from build123d import *

# Parameters (mm, degrees)
F1_DEPTH        = 1
F3_DEPTH        = 0.5
F5_DEPTH        = 5
F10_D           = 2
F10_DEPTH       = 5
F10_TIP         = 0.600860619
F10_ON_F7_D     = 2
F10_ON_F7_DEPTH = 5
F10_ON_F7_TIP   = 0.600860619
F10_ON_F8_D     = 2
F10_ON_F8_DEPTH = 5
F10_ON_F8_TIP   = 0.600860619
F10_ON_F9_D     = 2
F10_ON_F9_DEPTH = 5
F10_ON_F9_TIP   = 0.600860619


# Not quite as in the source:
# - ends of sketch curves that miss each other by under 0.0002 mm in the source are joined


with BuildPart() as f1:
    # F0 (on Top) → F1 (new body)
    with BuildSketch(Plane.XY):
        with BuildLine():
            ThreePointArc((87.5, -67.5), (100, 0), (87.5, 67.5))
            ThreePointArc((87.5, 67.5), (0, 75), (-87.5, 67.5))
            ThreePointArc((-87.5, 67.5), (-100, 0), (-87.5, -67.5))
            ThreePointArc((-87.5, -67.5), (0, -75), (87.5, -67.5))
        make_face()
    extrude(amount=F1_DEPTH)

    # F2 (on face) → F3 (cut)
    with BuildSketch(Plane(origin=(0, 0, 0), x_dir=(1, 0, 0), z_dir=(0, 0, -1))):
        Polygon((59.9405638027, -1.5313209672), (59.9405638027, -3.714e-05), (59.9405638027, 1.5331036891), (59.6300730728, 6.1295549733), (58.7212563071, 12.0819890983), (57.2441969375, 17.8245820004), (55.2293497966, 23.3313356518), (52.7045699138, 28.5721666207), (49.7021691234, 33.5132774711), (46.2529736583, 38.1275559743), (42.3840957472, 42.3849186981), (38.126361623, 46.2537966092), (33.5117117195, 49.7033634747), (28.5691152675, 52.705764265), (23.3301413005, 55.2305441479), (17.8233876491, 57.2453912888), (12.078937745, 58.7224506584), (6.1268750204, 59.6308960237), (1.5300523358, 59.9395297516), (-0.0008600909, 59.9395297516), (-1.5343723204, 59.9395297516), (-6.1304522042, 59.6308960237), (-12.0828863293, 58.7224506584), (-17.8277076337, 57.2453912888), (-23.3344612852, 55.2305441479), (-28.5734352521, 52.705764265), (-33.5160317041, 49.7033634747), (-38.1304216273, 46.2537966092), (-42.3860387693, 42.3849186981), (-46.2548052603, 38.1275559743), (-49.7044464059, 33.5132774711), (-52.7068100562, 28.5721666207), (-55.2315527989, 23.3313356518), (-57.24651136, 17.8245820004), (-58.7234964495, 12.0819890983), (-59.6322389351, 6.1295549733), (-59.9405384027, 1.5331036891), (-59.9405384027, -3.714e-05), (-59.9405384027, -1.5313209672), (-59.6322389351, -6.127400851), (-58.7234964495, -12.079834976), (-57.24651136, -17.8246562804), (-55.2315527989, -23.3314099319), (-52.7068100562, -28.5722409008), (-49.7044464059, -33.5130917709), (-46.2548052603, -38.1273702741), (-42.3860387693, -42.3850672583), (-38.1284160652, -46.251753907), (-33.5141747021, -49.7034748948), (-28.5734352521, -52.705764265), (-23.3326042832, -55.2285014457), (-17.8254792313, -57.2434600068), (-12.0828863293, -58.7204450962), (-6.1304522042, -59.6291875818), (-1.5343723204, -59.9395297516), (-0.0008600909, -59.9395297516), (1.5300523358, -59.9395297516), (6.1268750204, -59.6291875818), (12.078937745, -58.7204450962), (17.8233876491, -57.2434600068), (23.3301413005, -55.2285014457), (28.5691152675, -52.705764265), (33.5117117195, -49.7034748948), (38.126361623, -46.251753907), (42.3840957472, -42.3850672583), (46.2529736583, -38.1273702741), (49.7021691234, -33.5130917709), (52.7045699138, -28.5722409008), (55.2293497966, -23.3314099319), (57.2441969375, -17.8246562804), (58.7212563071, -12.079834976), (59.6300730728, -6.127400851), align=None)
        Polygon((38.1304470273, -28.6145805458), (15.9292456364, -35.0243199768), (0.9922645644, 2.8311480684), (-20.9062448628, -31.6715753619), (-34.6344668525, -31.6715771942), (-4.051352795, 17.7139046828), (-7.4845780431, 27.4743070541), (-19.3931602971, 27.4743070541), (-19.3931602971, 39.1043390122), (0.9922645644, 39.1043390122), (24.4064596442, -20.4359724552), (34.6987073808, -17.08074129), align=None, mode=Mode.SUBTRACT)
    extrude(amount=-F3_DEPTH, mode=Mode.SUBTRACT)

    # F4 (on face) → F5 (join)
    with BuildSketch(Plane.XY.offset(1)):
        with BuildLine():
            ThreePointArc((-24.5, -31.5), (-26.267766953, -32.232233047), (-27, -34))
            Line((-27, -34), (-24.5, -34))
            Line((-24.5, -34), (-24.5, -31.5))
        make_face()
        with BuildLine():
            Line((-24.5, -31.5), (-24.5, -34))
            Line((-24.5, -34), (-22, -34))
            ThreePointArc((-22, -34), (-22.732233047, -32.232233047), (-24.5, -31.5))
        make_face()
        with BuildLine():
            Line((-22, -34), (-24.5, -34))
            Line((-24.5, -34), (-24.5, -36.5))
            ThreePointArc((-24.5, -36.5), (-22.732233047, -35.767766953), (-22, -34))
        make_face()
        with BuildLine():
            Line((-24.5, -34), (-27, -34))
            ThreePointArc((-27, -34), (-26.267766953, -35.767766953), (-24.5, -36.5))
            Line((-24.5, -36.5), (-24.5, -34))
        make_face()
        with BuildLine():
            Line((-24.5, 24), (-24.5, 26.5))
            ThreePointArc((-24.5, 26.5), (-26.267766953, 25.767766953), (-27, 24))
            Line((-27, 24), (-24.5, 24))
        make_face()
        with BuildLine():
            Line((-24.5, 24), (-27, 24))
            ThreePointArc((-27, 24), (-26.267766953, 22.232233047), (-24.5, 21.5))
            Line((-24.5, 21.5), (-24.5, 24))
        make_face()
        with BuildLine():
            ThreePointArc((-22, 24), (-22.732233047, 25.767766953), (-24.5, 26.5))
            Line((-24.5, 26.5), (-24.5, 24))
            Line((-24.5, 24), (-22, 24))
        make_face()
        with BuildLine():
            Line((-22, 24), (-24.5, 24))
            Line((-24.5, 24), (-24.5, 21.5))
            ThreePointArc((-24.5, 21.5), (-22.732233047, 22.232233047), (-22, 24))
        make_face()
        with BuildLine():
            Line((24.5, -34), (24.5, -31.5))
            ThreePointArc((24.5, -31.5), (22.732233047, -32.232233047), (22, -34))
            Line((22, -34), (24.5, -34))
        make_face()
        with BuildLine():
            ThreePointArc((22, -34), (22.732233047, -35.767766953), (24.5, -36.5))
            Line((24.5, -36.5), (24.5, -34))
            Line((24.5, -34), (22, -34))
        make_face()
        with BuildLine():
            Line((24.5, -34), (27, -34))
            ThreePointArc((27, -34), (26.267766953, -32.232233047), (24.5, -31.5))
            Line((24.5, -31.5), (24.5, -34))
        make_face()
        with BuildLine():
            ThreePointArc((24.5, -36.5), (26.267766953, -35.767766953), (27, -34))
            Line((27, -34), (24.5, -34))
            Line((24.5, -34), (24.5, -36.5))
        make_face()
        with BuildLine():
            Line((24.5, 24), (24.5, 26.5))
            ThreePointArc((24.5, 26.5), (22.732233047, 25.767766953), (22, 24))
            Line((22, 24), (24.5, 24))
        make_face()
        with BuildLine():
            ThreePointArc((27, 24), (26.267766953, 25.767766953), (24.5, 26.5))
            Line((24.5, 26.5), (24.5, 24))
            Line((24.5, 24), (27, 24))
        make_face()
        with BuildLine():
            Line((27, 24), (24.5, 24))
            Line((24.5, 24), (24.5, 21.5))
            ThreePointArc((24.5, 21.5), (26.267766953, 22.232233047), (27, 24))
        make_face()
        with BuildLine():
            Line((24.5, 21.5), (24.5, 24))
            Line((24.5, 24), (22, 24))
            ThreePointArc((22, 24), (22.732233047, 22.232233047), (24.5, 21.5))
        make_face()
    extrude(amount=F5_DEPTH)

    # F10
    with Locations(Plane.XY.offset(6)):
        with Locations((-24.5, 24)):
            Hole(F10_D / 2, depth=F10_DEPTH)
            with Locations((0, 0, -(F10_DEPTH + F10_TIP / 2))):  # 118° drill point
                Cone(0, F10_D / 2, F10_TIP, mode=Mode.SUBTRACT)

    # F10 on F7
    with Locations(Plane.XY.offset(6)):
        with Locations((24.5, 24)):
            Hole(F10_ON_F7_D / 2, depth=F10_ON_F7_DEPTH)
            with Locations((0, 0, -(F10_ON_F7_DEPTH + F10_ON_F7_TIP / 2))):  # 118° drill point
                Cone(0, F10_ON_F7_D / 2, F10_ON_F7_TIP, mode=Mode.SUBTRACT)

    # F10 on F8
    with Locations(Plane.XY.offset(6)):
        with Locations((-24.5, -34)):
            Hole(F10_ON_F8_D / 2, depth=F10_ON_F8_DEPTH)
            with Locations((0, 0, -(F10_ON_F8_DEPTH + F10_ON_F8_TIP / 2))):  # 118° drill point
                Cone(0, F10_ON_F8_D / 2, F10_ON_F8_TIP, mode=Mode.SUBTRACT)

    # F10 on F9
    with Locations(Plane.XY.offset(6)):
        with Locations((24.5, -34)):
            Hole(F10_ON_F9_D / 2, depth=F10_ON_F9_DEPTH)
            with Locations((0, 0, -(F10_ON_F9_DEPTH + F10_ON_F9_TIP / 2))):  # 118° drill point
                Cone(0, F10_ON_F9_D / 2, F10_ON_F9_TIP, mode=Mode.SUBTRACT)


solid = f1.part
Work out the finished part from the listing and answer in its coordinate system (mm). A direction names the side the tool comes from. Coordinates: 2 decimals unless noted, no trailing zeros. Write each loop counter-clockwise with the first axis right and the second up, starting at its lowest first coordinate (ties: lowest second). Pieces come first, ordered by that corner, then holes. Notation, with made-up numbers: M -1,89 L 58,89 A22 ccw 58,113 Z; hole C 52.5,-23.5 d3. An arc over 180 degrees is marked long. Use one line per item in the form item = value. Start each with the question number.
1. Each of these flat-tipped pins is pushed along its axis until it touches: P1, Ø6, axis at x = -19, y = 37.5, coming from the -Z side; P2, Ø0.6, axis at y = -33.5, z = 0, coming from the -X side; P3, Ø1.2, axis at x = -24.5, y = 24, coming from the +Z side. Where does it stop, or does it pass through?
2. The part is cut by section A-A (z = 2). Give the vertices of the cut face in (x, y), plus the area to 3 significant figures.
3. The part is cut by section B-B (y = 9.5). Give the vertices of the cut face in (x, z).
4. A tool of negligible diameter and unlimited length cuts with its end or side. For faces 1 (the face through (-23, -34, 6)), 2 (the face through (-44.29, -40.29, 0.25)), from which of +Z, -Z, +X, -X, +Y, -Y can it reach the whole face along a straight path? Write none if from no direction.
5. Straight lines are drawn through the part: probe 1 along Y at (x, z) = (-24.5, 4.9); probe 2 along X at (y, z) = (-34, 5); probe 3 along Z at (x, y) = (29.5, 15.5). For each, find the intervals that lie inside material, in ascending order. Write a range as from..to.
Evaluation:
q1.P1 = 0.5
q1.P2 = -97.05
q1.P3 = 0.76
q2.outline = C -24.5,-34 d5; C -24.5,24 d5; C 24.5,-34 d5; C 24.5,24 d5; hole C -24.5,-34 d2; hole C -24.5,24 d2; hole C 24.5,-34 d2; hole C 24.5,24 d2
q2.area = 66.0 mm^2
q3.outline = M -99.76,0 L -59.12,0 L -59.12,0.5 L -20.9,0.5 L -20.9,0 L -6.83,0 L -6.83,0.5 L 5.86,0.5 L 5.86,0 L 20.11,0 L 20.11,0.5 L 59.12,0.5 L 59.12,0 L 99.76,0 L 99.76,1 L -99.76,1 Z
q4.face_1 = +Z, +X, -X, +Y, -Y
q4.face_2 = -Z
q5.probe_1 = -36.5..-35, -33..-31.5, 21.5..23, 25..26.5
q5.probe_2 = -27..-25.5, -23.5..-22, 22..23.5, 25.5..27
q5.probe_3 = 0.5..1
